Could you check a few things on this model? Use its own coordinates, in mm. A direction names the side the tool comes from. Round coordinates to 2 decimals unless told otherwise and drop trailing zeros. Write each loop counter-clockwise with the first axis right and the second up, starting at its lowest first coordinate (ties: lowest second). Pieces come first, ordered by that corner, then holes. Notation, with made-up numbers: (82, 76.5) - (118, 76.5) arc R34 cw to (118, 109.5) - close; hole circle Ø3 at (-23, 78). An arc over 180 degrees is marked (long way). Write each question's results on one line, items separated by ' | '. Start each with the question number.
(1) Imagine slicing it at D-D on z = -78.5. Write out the boundary of the cut face in (x, y), then the cut area to 3 significant figures.
(2) Please list where these lines run through material, in increasing order: line 1 (Z direction, x = -162.5, y = -6); line 2 (Z direction, x = -45.5, y = 0.75); line 3 (X direction, y = -2, z = -139.5). Write a range as [from, to].
(3) For P1, Ø7, axis at x = -168, y = -4, coming from the -Z side; P2, Ø5, axis at y = -3, z = -22, coming from the +X side; P3, Ø4, axis at y = -4, z = -139.5, coming from the -X side; P4, Ø3, axis at y = -2.5, z = -92.5, coming from the -X side, each with a flat end and sliding along its axis, tell me the tip position at first contact or that it passes through.
(4) Imagine slicing it at C-C on z = -20.5. Write out the boundary of the cut face in (x, y).
(5) On a 3-axis mill with a long thin cutter (end or side, diameter ignored), from which of +Z, -Z, +X, -X, +Y, -Y can I reach the whole of each face in a straight line? I mean faces 1 (the flat face through (-152.4, -6, -143)), 2 (the flat face through (-165.1, -6, -133)), 3 (the flat face through (-29, 3, -25.4)), 4 (the flat face through (-16, -6, -146.05)). Say none if no direction works.
(6) Thinking about a two-plate mould opening in Z: for faces 5 (the flat face through (-171.45, -6, -16)), 6 (the flat face through (-29, 3, -44.45)), 7 (the flat face through (-90, 3, -152.4)), which applies, +Z half, -Z half, draft (parallel to the pull), parting line (faces both ways), or undercut?
(7) Imagine slicing it at A-A on y = -2. Write out the boundary of the cut face in (x, z), then the cut area to 3 significant figures.
(8) Imagine slicing it at B-B on x = -15. Write out the boundary of the cut face in (y, z).
```python
from build123d import *

# Parameters (mm, degrees)
SKETCH1_W           = 177.8
SKETCH1_H           = 152.4
SKETCH1_W_2         = 44.45
SKETCH1_H_2         = 19.05
BOSS_EXTRUDE1_DEPTH = 6.35
BOSS_EXTRUDE2_DEPTH = 12.7


with BuildPart() as part:
    # Sketch1 → Boss-Extrude1 (new body)
    with BuildSketch(Plane(origin=(0, 0, 0), x_dir=(1, 0, 0), z_dir=(0, 1, 0))):
        with Locations((-88.9, 76.2)):
            Rectangle(SKETCH1_W, SKETCH1_H)
        with Locations((-28.575, 34.925)):
            Rectangle(SKETCH1_W_2, SKETCH1_H_2, mode=Mode.SUBTRACT)
    extrude(amount=BOSS_EXTRUDE1_DEPTH)

    # Sketch2 → Boss-Extrude2 (add)
    with BuildSketch(Plane.XZ):
        Polygon((-171.45, -146.05), (-171.45, -127), (-165.1, -127), (-165.1, -139.720102982), (-152.4, -139.720102982), (-152.4, -146.05), align=None)
        Polygon((-6.35, -146.05), (-25.4, -146.05), (-25.4, -139.720102982), (-12.7, -139.720102982), (-12.7, -127), (-6.35, -127), align=None)
        Polygon((-171.45, -6.35), (-152.4, -6.35), (-152.4, -12.7), (-165.1, -12.7), (-165.1, -25.4), (-171.45, -25.4), align=None)
    extrude(amount=BOSS_EXTRUDE2_DEPTH)


solid = part.part
```
Response:
1) outline: (-177.8, 0) - (0, 0) - (0, 6.35) - (-177.8, 6.35) - close | area: 1,130 mm²
2) line 1: [-146.05, -139.72], [-12.7, -6.35] | line 2: [-152.4, -44.45], [-25.4, 0] | line 3: [-171.45, -165.1], [-12.7, -6.35]
3) P1: z = -146.05 | P2: x = -165.1 | P3: x = -171.45 | P4: through
4) outline: (-177.8, 0) - (-171.45, 0) - (-171.45, -12.7) - (-165.1, -12.7) - (-165.1, 0) - (0, 0) - (0, 6.35) - (-177.8, 6.35) - close
5) face 1: +Z, -Z, -Y | face 2: -Y | face 3: +Y, -Y | face 4: -Z, +X, -X, -Y
6) face 5: draft | face 6: undercut | face 7: -Z half
7) outline: (-171.45, -146.05) - (-152.4, -146.05) - (-152.4, -139.72) - (-165.1, -139.72) - (-165.1, -127) - (-171.45, -127) - close; (-171.45, -25.4) - (-165.1, -25.4) - (-165.1, -12.7) - (-152.4, -12.7) - (-152.4, -6.35) - (-171.45, -6.35) - close; (-25.4, -146.05) - (-6.35, -146.05) - (-6.35, -127) - (-12.7, -127) - (-12.7, -139.72) - (-25.4, -139.72) - close | area: 604 mm²
8) outline: (-12.7, -146.05) - (0, -146.05) - (0, -152.4) - (6.35, -152.4) - (6.35, -44.45) - (0, -44.45) - (0, -139.72) - (-12.7, -139.72) - close; (0, -25.4) - (6.35, -25.4) - (6.35, 0) - (0, 0) - close
